```python
from build123d import *

# Parameters (mm, degrees)
SKETCH1_R           = 1.75
BOSS_EXTRUDE1_DEPTH = 8
SKETCH2_W           = 46
SKETCH2_H           = 21
CUT_EXTRUDE1_DEPTH  = 2
SKETCH3_R           = 1
CUT_EXTRUDE2_DEPTH  = 2
CUT_EXTRUDE3_DEPTH  = 6
SKETCH5_W           = 10.927537962
SKETCH5_H           = 9.870451426
CUT_EXTRUDE4_DEPTH  = 7
FILLET4_R           = 6
CHAMFER2_SIZE       = 1
SKETCH7_R           = 2
BOSS_EXTRUDE2_DEPTH = 2
FILLET5_R           = 1


with BuildPart() as part:
    # Sketch1 → Boss-Extrude1 (new body)
    with BuildSketch(Plane.XY):
        with BuildLine():
            Line((-4.75, -42), (-4.75, -39))
            Line((-4.75, -39), (-25, -39))
            Line((-25, -39), (-25, 0))
            Line((-25, 0), (25, 0))
            Line((25, 0), (25, -39))
            Line((25, -39), (4.75, -39))
            Line((4.75, -39), (4.75, -42))
            ThreePointArc((4.75, -42), (0, -46.75), (-4.75, -42))
        make_face()
        with Locations((-20, -5)):
            Circle(SKETCH1_R, mode=Mode.SUBTRACT)
        with Locations((20, -5)):
            Circle(SKETCH1_R, mode=Mode.SUBTRACT)
        with Locations((0, -42)):
            Circle(SKETCH1_R, mode=Mode.SUBTRACT)
    extrude(amount=BOSS_EXTRUDE1_DEPTH)

    # Sketch2 → Cut-Extrude1 (cut)
    with BuildSketch(Plane.XY.offset(8)):
        with Locations((0, -26.5)):
            Rectangle(SKETCH2_W, SKETCH2_H)
    extrude(amount=-CUT_EXTRUDE1_DEPTH, mode=Mode.SUBTRACT)

    # Sketch3 → Cut-Extrude2 (cut)
    with BuildSketch(Plane.XY.offset(6)):
        with Locations((-20.45, -18.3)):
            Circle(SKETCH3_R)
        with Locations((20.45, -18.3)):
            Circle(SKETCH3_R)
        with Locations((20.45, -34.7)):
            Circle(SKETCH3_R)
        with Locations((-20.45, -34.7)):
            Circle(SKETCH3_R)
        with BuildLine():
            Line((-17.95, -18.3), (-17.95, -16))
            Line((-17.95, -16), (17.95, -16))
            Line((17.95, -16), (17.95, -18.3))
            ThreePointArc((17.95, -18.3), (18.682233047, -20.067766953), (20.45, -20.8))
            Line((20.45, -20.8), (23, -20.8))
            Line((23, -20.8), (23, -32.2))
            Line((23, -32.2), (20.45, -32.2))
            ThreePointArc((20.45, -32.2), (18.682233047, -32.932233047), (17.95, -34.7))
            Line((17.95, -34.7), (17.95, -37))
            Line((17.95, -37), (-17.95, -37))
            Line((-17.95, -37), (-17.95, -34.7))
            ThreePointArc((-17.95, -34.7), (-18.682233047, -32.932233047), (-20.45, -32.2))
            Line((-20.45, -32.2), (-23, -32.2))
            Line((-23, -32.2), (-23, -20.8))
            Line((-23, -20.8), (-20.45, -20.8))
            ThreePointArc((-20.45, -20.8), (-18.682233047, -20.067766953), (-17.95, -18.3))
        make_face()
    extrude(amount=-CUT_EXTRUDE2_DEPTH, mode=Mode.SUBTRACT)

    # Sketch4 → Cut-Extrude3 (cut)
    with BuildSketch(Plane.XY.offset(8)):
        Polygon((-7.723, 0), (-7.723, -6.1725), (-6.723, -7.1725), (-6.723, -17.5725), (6.723, -17.5725), (6.723, -7.1725), (7.723, -6.1725), (7.723, 0), align=None)
    extrude(amount=-CUT_EXTRUDE3_DEPTH, mode=Mode.SUBTRACT)

    # Sketch5 → Cut-Extrude4 (cut)
    with BuildSketch(Plane.XY.offset(8)):
        with Locations((0, -15.479727473)):
            Rectangle(SKETCH5_W, SKETCH5_H)
    extrude(amount=-CUT_EXTRUDE4_DEPTH, mode=Mode.SUBTRACT)

    # Fillet4
    fillet4_edges = [part.edges().sort_by_distance(p)[0] for p in [
        (25, -39, 4),
        (4.75, -39, 4),
        (-25, -39, 4),
        (-4.75, -39, 4),
        (25, 0, 4),
        (-25, 0, 4),
    ]]
    fillet(fillet4_edges, radius=FILLET4_R)

    # Chamfer2
    chamfer2_edges = [part.edges().sort_by_distance(p)[0] for p in [
        (-1.75, -42, 0),
        (-21.75, -5, 0),
        (18.25, -5, 0),
    ]]
    chamfer(chamfer2_edges, length=CHAMFER2_SIZE)

    # Sketch7 → Boss-Extrude2 (add)
    with BuildSketch(Plane(origin=(0, 0, 0), x_dir=(-1, 0, 0), z_dir=(0, 0, -1))):
        with BuildLine():
            Line((-25, -14.5), (-30, -14.5))
            ThreePointArc((-30, -14.5), (-35, -19.5), (-30, -24.5))
            Line((-30, -24.5), (-25, -24.5))
            Line((-25, -24.5), (-25, -14.5))
        make_face()
        with Locations((-30, -19.5)):
            Circle(SKETCH7_R, mode=Mode.SUBTRACT)
        with BuildLine():
            Line((30, -14.5), (25, -14.5))
            Line((25, -14.5), (25, -24.5))
            Line((25, -24.5), (30, -24.5))
            ThreePointArc((30, -24.5), (35, -19.5), (30, -14.5))
        make_face()
        with Locations((30, -19.5)):
            Circle(SKETCH7_R, mode=Mode.SUBTRACT)
    extrude(amount=-BOSS_EXTRUDE2_DEPTH)

    # Fillet5
    fillet5_edges = [part.edges().sort_by_distance(p)[0] for p in [
        (25, -14.5, 1),
        (25, -24.5, 1),
        (25, -19.5, 2),
        (-25, -24.5, 1),
        (-25, -14.5, 1),
        (-25, -19.5, 2),
    ]]
    fillet(fillet5_edges, radius=FILLET5_R)


solid = part.part
```
Geometry: final body of the model. Coordinates: model frame, mm. A direction names the side the tool comes from. Round coordinates to 2 decimals unless told otherwise and drop trailing zeros. Order: outer loops, then holes, each group sorted by start corner. A loop starts at its lowest first (then second) coordinate and runs counter-clockwise, first axis right, second up. Notation, with made-up numbers: (54.25, 47.5) -> (112.25, 47.5) arc R28 ccw to (112.25, 75.5) -> close; hole circle Ø9 at (-34, 32.25). An arc over 180 degrees is marked (long way). Use one line per item in the form item = value.
(1) First-contact query: pin 1 Ø2 at (x, y) = (20, -18) entering from +Z; pin 2 Ø3 at (x, y) = (19.5, -22.5) entering from -Z; pin 3 Ø1.5 at (x, y) = (0, -5) entering from +Z; pin 4 Ø1.6 at (x, z) = (-22, 5) entering from -Y. Flat tips, straight axial feed; report the tip coordinate or a pass-through.
Results list:
pin_1 = 6
pin_2 = 0
pin_3 = 2
pin_4 = -38.58
(2) Draft query along X for faces 4 (the face through (-30, -22, 2)), 5 (the face through (0, -15, 1)), 6 (the face through (25, -19, 5)). Return one class per face: pulls with the +X half, pulls with the -X half, needs draft (parallel to the pull), parting line crosses it, or undercut.
Results list:
face_4 = needs draft
face_5 = undercut
face_6 = pulls with the +X half
(3) Section A-A on x = 0. Return loops of the section in (y, z).
Results list:
outline = (-46.75, 0) -> (-44.75, 0) -> (-43.75, 1) -> (-43.75, 8) -> (-46.75, 8) -> close; (-40.25, 1) -> (-39.25, 0) -> (0, 0) -> (0, 2) -> (-10.54, 2) -> (-10.54, 1) -> (-20.41, 1) -> (-20.41, 4) -> (-37, 4) -> (-37, 8) -> (-40.25, 8) -> close
(4) Section C-C on z = 7.25. Count the separate pieces of the cut face and the enclosed holes in it, and give its area (3 significant figures).
Results list:
separate_pieces = 1
enclosed_holes = 3
area = 771 mm^2
(5) Ray query, probe 1 along Y at (x, z) = (30, 0.9); probe 2 along Y at (x, z) = (20.45, 4.6); probe 3 along X at (y, z) = (-8, 6). Return the intervals inside material, ascending. Write a range as [from, to].
Results list:
probe_1 = [-24.5, -21.5], [-17.5, -14.5]
probe_2 = [-38.82, -35.7], [-33.7, -32.2], [-20.8, -19.3], [-17.3, -6.69], [-3.31, -0.18]
probe_3 = [-25, -6.72], [6.72, 25]
(6) Access query for faces 1 (the face through (6.723, -12, 5)), 2 (the face through (-28, -24.5, 1)), 3 (the face through (18.663, -20.048, 5.014)). Directions: +Z, -Z, +X, -X, +Y, -Y. A direction counts if a zero-diameter tool reaches every point of the face in a straight line with its end or side. Return the directions, or none.
Results list:
face_1 = +Z, +Y
face_2 = +Z, -Z, -X, -Y
face_3 = +Z
(7) Section B-B on y = -23.5. Return loops of the section in (x, z).
Results list:
outline = (-33, 0) -> (33, 0) -> (33, 2) -> (26, 2) arc R1 cw to (25, 3) -> (25, 8) -> (23, 8) -> (23, 4) -> (-23, 4) -> (-23, 8) -> (-25, 8) -> (-25, 3) arc R1 cw to (-26, 2) -> (-33, 2) -> close
